CAD build for the part. Positions are in the model's coordinates, mm. Face numbers are marked on the shaded views. Round coordinates to 2 decimals unless told otherwise and drop trailing zeros. Order: outer loops, then holes, each group sorted by start corner. A loop starts at its lowest first (then second) coordinate and runs counter-clockwise, first axis right, second up. Notation, with made-up numbers: M 82,80 L 100,80 A18 ccw 100,108 Z; hole C -15.75,46 d7. An arc over 180 degrees is marked long. Answer as a JSON object with one key per item and string values.
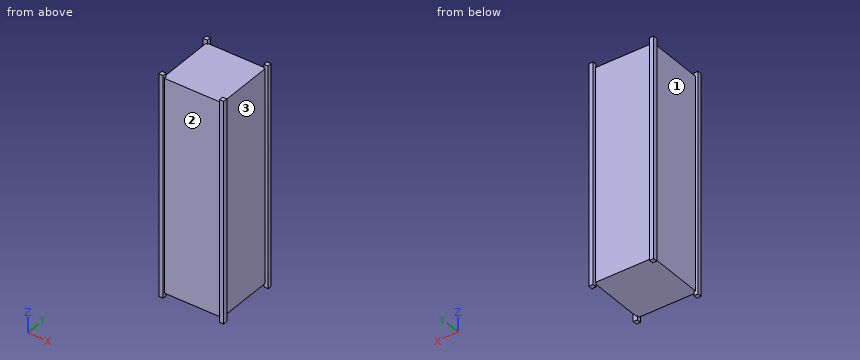
```python
from build123d import *

# Parameters (mm, degrees)
SKETCH1_W             = 6.5
SKETCH1_H             = 6.5
BOSS_EXTRUDE1_DEPTH   = 340.5
BOSS_EXTRUDE1_2_DEPTH = 340.5
BOSS_EXTRUDE1_3_DEPTH = 340.5
BOSS_EXTRUDE1_4_DEPTH = 340.5
SKETCH2_W             = 91.305836421
SKETCH2_H             = 92.06883784
BOSS_EXTRUDE2_DEPTH   = 328.5


with BuildPart() as part:
    # Sketch1 → Boss-Extrude1 (new body)
    with BuildSketch(Plane.XY):
        with Locations((3.25, 96.75)):
            Rectangle(SKETCH1_W, SKETCH1_H)
    extrude(amount=-BOSS_EXTRUDE1_DEPTH)



with BuildPart() as body_2:
    # Sketch1 → Boss-Extrude1 2 (new body)
    with BuildSketch(Plane.XY):
        with Locations((96.75, 96.75)):
            Rectangle(SKETCH1_W, SKETCH1_H)
    extrude(amount=-BOSS_EXTRUDE1_2_DEPTH)


with BuildPart() as body_3:
    # Sketch1 → Boss-Extrude1 3 (new body)
    with BuildSketch(Plane.XY):
        with Locations((96.75, 3.25)):
            Rectangle(SKETCH1_W, SKETCH1_H)
    extrude(amount=-BOSS_EXTRUDE1_3_DEPTH)


with BuildPart() as body_4:
    # Sketch1 → Boss-Extrude1 4 (new body)
    with BuildSketch(Plane.XY):
        with Locations((3.25, 3.25)):
            Rectangle(SKETCH1_W, SKETCH1_H)
    extrude(amount=-BOSS_EXTRUDE1_4_DEPTH)


with BuildPart() as part_1:
    add(part.part)

    add(body_2.part)  # Boss-Extrude2 merges body 2

    add(body_3.part)  # Boss-Extrude2 merges body 3

    add(body_4.part)  # Boss-Extrude2 merges body 4
    # Sketch2 → Boss-Extrude2 (add)
    with BuildSketch(Plane(origin=(0, 0, -6), x_dir=(-1, 0, 0), z_dir=(0, 0, -1))):
        with Locations((-49.653832388, 49.017997872)):
            Rectangle(SKETCH2_W, SKETCH2_H)
    extrude(amount=BOSS_EXTRUDE2_DEPTH)


solid = part_1.part
```
Item 1: Saw through at B-B on y = 72.5. List the corners of the cut face in (x, z), and give its area (3 significant figures).
Worked answers:
{"outline": "M 4,-334.5 L 95.31,-334.5 L 95.31,-6 L 4,-6 Z", "area": "30,000 mm2"}
Item 2: Saw through at A-A on z = -149. List the corners of the cut face in (x, y).
Worked answers:
{"outline": "M 0,0 L 6.5,0 L 6.5,2.98 L 93.5,2.98 L 93.5,0 L 100,0 L 100,6.5 L 95.31,6.5 L 95.31,93.5 L 100,93.5 L 100,100 L 93.5,100 L 93.5,95.05 L 6.5,95.05 L 6.5,100 L 0,100 L 0,93.5 L 4,93.5 L 4,6.5 L 0,6.5 Z"}
Item 3: Wall check: line 1 along Y through (x, z) = (89, -179); line 2 along X through (y, z) = (13, -137.5); line 3 along Z through (x, y) = (13.5, 38). Give the ranges that are in metal, low to high. Write a range as [from, to].
Worked answers:
{"line 1": "y = [2.98, 95.05]", "line 2": "x = [4, 95.31]", "line 3": "z = [-334.5, -6]"}
Item 4: Saw through at C-C on x = 57. List the corners of the cut face in (y, z).
Worked answers:
{"outline": "M 2.98,-334.5 L 95.05,-334.5 L 95.05,-6 L 2.98,-6 Z"}
Item 5: Two-plate mould, pull along X, no slides. Class the marked faces 1, 2 and 3: released by +X, released by -X, zero draft, split by the parting line, or undercut.
Worked answers:
{"face 1": "released by -X", "face 2": "undercut", "face 3": "released by +X"}
Item 6: Drop flat-ended pins along their axis: pin 1 Ø10 at (x, y) = (59, 17.5) entering from -Z; pin 2 Ø2 at (x, y) = (27.5, 44) entering from +Z; pin 3 Ø3 at (y, z) = (63.5, -94.5) entering from +X; pin 4 Ø7 at (y, z) = (96, -130.5) entering from -X. Give the stop position or say it passes through.
Worked answers:
{"pin 1": "stops at z = -334.5", "pin 2": "stops at z = -6", "pin 3": "stops at x = 95.31", "pin 4": "stops at x = 0"}
